Input: dimensioned drawing with shaded views. Units: mm. Origin: part minimum x, y, z. A direction names the side the tool comes from. Round coordinates to 2 decimals unless told otherwise and drop trailing zeros. Write each loop counter-clockwise with the first axis right and the second up, starting at its lowest first coordinate (ties: lowest second). Pieces come first, ordered by that corner, then holes. Notation, with made-up numbers: (56, 70) -> (90, 70) arc R20 cw to (90, 78) -> close; hole circle Ø3 at (12.5, 26.5). An arc over 180 degrees is marked (long way). One line per item, written item: value. Start each with the question number.
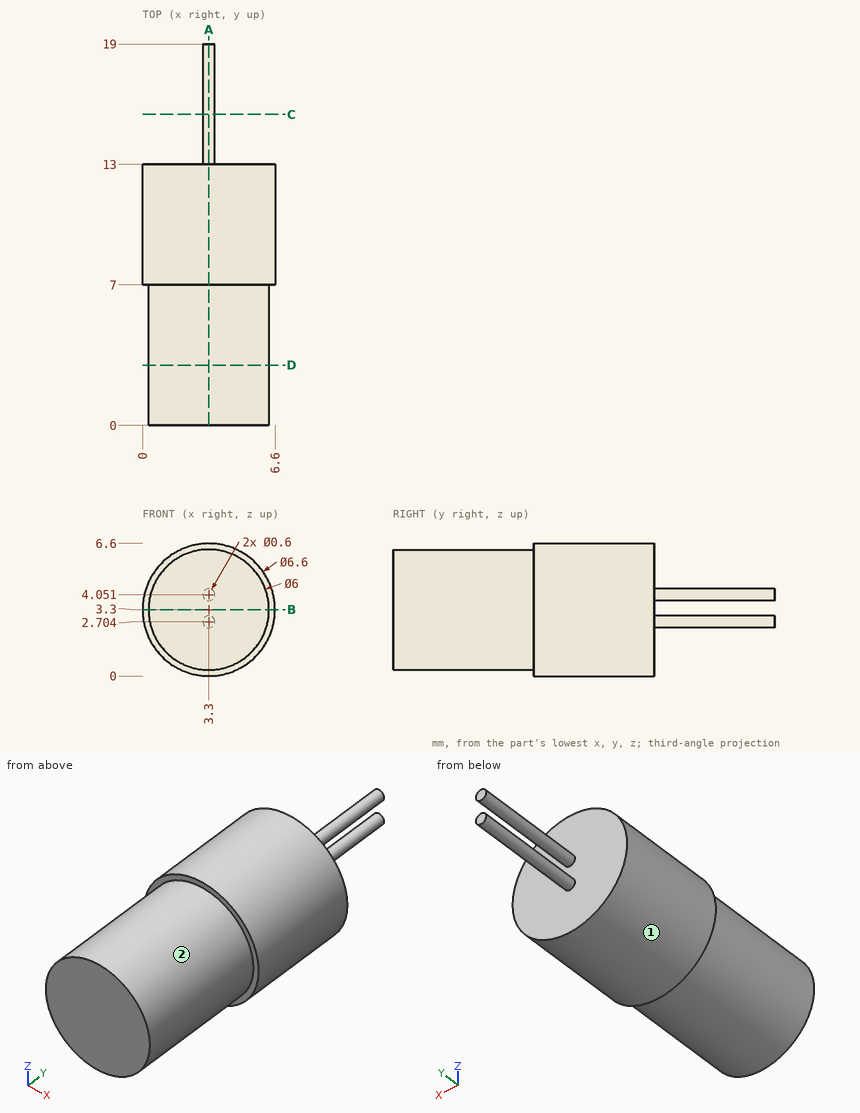
(1) Section query C-C (y = 15.5). Output: boundary loops of the cut face in (x, z).
(2) Pin query (flat end, axial travel): pin 1 (3 mm diameter, centred on y = 8.5, z = 5, fed in from -X); pin 2 (1 mm diameter, centred on x = 4, y = 5, fed in from +Z). Return the tip coordinate at first contact, or that it passes through.
(3) Section query A-A (x = 3.3). Output: boundary loops of the cut face in (y, z).
(4) Line query: probe 1 along Y at (x, z) = (2, 3.5); probe 2 along Y at (x, z) = (5.25, 5.75); probe 3 along Z at (x, y) = (1.25, 11) (1 decimal). Output: solid intervals per line, ascending.
(5) Section query D-D (y = 3). Output: boundary loops of the cut face in (x, z), and give its area (3 significant figures).
(6) Set-up query: the marked faces 1 and 2. Return all of +Z, -Z, +X, -X, +Y, -Y with unobstructed straight access to the full face (end or side cutting, diameter ignored); none if empty.
(7) Section query B-B (z = 3.3). Output: boundary loops of the cut face in (x, y).
Results list:
1. outline: circle Ø0.6 at (3.3, 2.7); circle Ø0.6 at (3.3, 4.05)
2. pin 1: stops at x = 0.01
2. pin 2: stops at z = 6.29
3. outline: (0, 0.3) -> (7, 0.3) -> (7, 0) -> (13, 0) -> (13, 2.4) -> (19, 2.4) -> (19, 3) -> (13, 3) -> (13, 3.75) -> (19, 3.75) -> (19, 4.35) -> (13, 4.35) -> (13, 6.6) -> (7, 6.6) -> (7, 6.3) -> (0, 6.3) -> close
4. probe 1: y = 0 to 13
4. probe 2: y = 7 to 13
4. probe 3: z = 0.7 to 5.9
5. outline: circle Ø6 at (3.3, 3.3)
5. area: 28.3 mm^2
6. face 1: +Y, -Y
6. face 2: -Y
7. outline: (0, 7) -> (0.3, 7) -> (0.3, 0) -> (6.3, 0) -> (6.3, 7) -> (6.6, 7) -> (6.6, 13) -> (0, 13) -> close
